Can you work these out from the model? Positions are in its coordinate system, mm. Give positions to 0.01 mm unless a question says otherwise; leave off trailing zeros. Loops run counter-clockwise (first coordinate to the right, second up) from the corner with the lowest first, then second, coordinate; pieces in that order, holes last. Notation, with made-up numbers: M 4,64 L 30,64 A29 cw 30,88 Z; hole C 58.5,-28 d7. An arc over 180 degrees is marked long. Use CSV: the item, a comma, the result in double quotes.
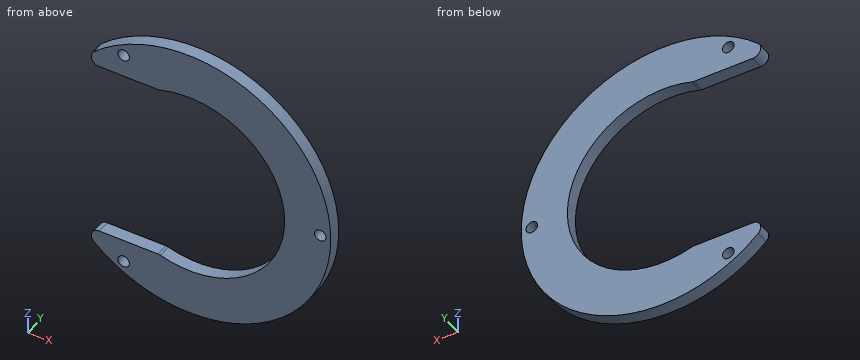
Autodesk Inventor part; units mm, degrees
ref_plane "YZ Plane" through (0, 0, 0) normal (1, 0, 0) x (0, 1, 0)
ref_plane "XZ Plane" through (0, 0, 0) normal (0, 1, 0) x (-1, 0, 0)
ref_plane "XY Plane" through (0, 0, 0) normal (0, 0, 1) x (1, 0, 0)
sketch "Sketch1" plane through (0, 0, 0) normal (0, 1, 0) x (-1, 0, 0)
  circle A0 centre (0, 0) radius 59
  circle A1 centre (0, 0) radius 81 construction
  circle A2 centre (0, 0) radius 87.5
  line L0 (90, -56) -> (10, -56)
  line L1 (10, -56) -> (10, 56)
  line L2 (10, 56) -> (90, 56)
  line L3 (90, 56) -> (90, -56)
  line L4 (90, -56) -> (10, 56) construction
  line L5 (10, -56) -> (90, 56) construction
  point P0 (50, 0)
  point P1 (90, 0)
  point P2 (10, 0)
  point P3 (60, -54.4151)
  point P4 (60, 54.4151)
  point P5 (80, 35.4436)
  point P6 (80, -35.4436)
  point P7 (67.2328, 56)
  point P8 (67.2328, -56)
  point P9 (18.5742, 56)
  point P10 (18.5742, -56)
  dimension "d0" = 118
  dimension "d1" = 162
  dimension "d2" = 175
  dimension "d7" = 112
  dimension "d9" = 80
  dimension "d10" = 10
extrude "Extrusion1" add sketch "Sketch1" along normal blind 8 contours A0 L0 A2 L2 picked at (48.009, -59.1067)
fillet "Fillet1" radius 5 4 edges at (-67.2328, 4, -56) (-67.2328, 4, 56) (-18.5742, 4, -56) (-18.5742, 4, 56)
sketch "Sketch2" plane through (0, 8, 0) normal (0, 1, 0) x (1, 0, 0)
  circle A0 centre (0, 0) radius 70.375
  line L0 (-36.4414, 79.1184) -> (-50.2978, 71.1184)
  line L1 (-50.2978, 71.1184) -> (-44.9056, 61.7788)
  arc A1 (-31.0492, 69.7788) -> (-44.9056, 61.7788) centre (0, 0) ccw
  line L2 (-31.0492, 69.7788) -> (-36.4414, 79.1184)
  circle A2 centre (-40.5, 70.1481) radius 3.5625
  circle A3 centre (-40.5, 70.1481) radius 3.5625
  line L3 (86.7392, -8) -> (86.7392, 8)
  line L4 (86.7392, 8) -> (75.9549, 8)
  arc A4 (75.9549, -8) -> (75.9549, 8) centre (0, 0) ccw
  line L5 (75.9549, -8) -> (86.7392, -8)
  arc A5 (80.9215, -3.5651) -> (80.9217, -3.5616) centre (0, 0) ccw
  arc A6 (81.0783, -3.5616) -> (80.9217, -3.5616) centre (81, 0) ccw
  line L6 (81.0783, -3.5616) -> (80.9215, -3.5651)
  line L7 (-50.2978, -71.1184) -> (-36.4414, -79.1184)
  line L8 (-36.4414, -79.1184) -> (-31.0492, -69.7788)
  arc A7 (-44.9056, -61.7788) -> (-31.0492, -69.7788) centre (0, 0) ccw
  line L9 (-44.9056, -61.7788) -> (-50.2978, -71.1184)
  circle A8 centre (-40.5, -70.1481) radius 3.5625
  point P0 (-65.1143, 450.6181)
extrude "Extrusion2" cut sketch "Sketch2" against normal blind 10 contours A2 | A5 A6 L6 | A8
properties part number "Cylinder Segment Holder" material "Acetal Resin, Black"
Q1. I want a section at C-C, the plane y = 4.25. State how many separate pieces and enclosed holes the cut face has, then the cut area to 3 significant figures.
Model answer:
separate pieces,"1"
enclosed holes,"3"
area,"9,250 mm2"
Q2. Please list where these lines run through material, in increasing order: L1, parallel to Z at x = 0, y = 4.75; L2, parallel to Z at x = -40.5, y = 4.25; L3, parallel to Z at x = -42, y = 5.5. Write a range as from..to.
Model answer:
L1,"-87.5..-59, 59..87.5"
L2,"-77.56..-73.71, -66.59..-56, 56..66.59, 73.71..77.56"
L3,"-76.76..-73.38, -66.92..-56, 56..66.92, 73.38..76.76"
Q3. I'm going to push flat-ended pins straight in: P1, Ø2, axis at y = 5, z = -31.5, coming from the +X side; P2, Ø2, axis at y = 1.5, z = 29, coming from the +X side; P3, Ø2, axis at y = 4.5, z = 58, coming from the +X side. Where does each tip first touch, or does it pass through?
Model answer:
P1,"x = 82.01"
P2,"x = 82.9"
P3,"x = 66.39"
Q4. I want a section at A-A, the plane x = 0. Please give me the cut outline in (y, z).
Model answer:
outline,"M 0,-87.5 L 8,-87.5 L 8,-59 L 0,-59 Z; M 0,59 L 8,59 L 8,87.5 L 0,87.5 Z"
Q5. I want a section at D-D, the plane x = -40.5. Please give me the cut outline in (y, z).
Model answer:
outline,"M 0,-77.56 L 8,-77.56 L 8,-73.71 L 0,-73.71 Z; M 0,-66.59 L 8,-66.59 L 8,-56 L 0,-56 Z; M 0,56 L 8,56 L 8,66.59 L 0,66.59 Z; M 0,73.71 L 8,73.71 L 8,77.56 L 0,77.56 Z"
Q6. I want a section at B-B, the plane z = 0. Please give me the cut outline in (x, y), then the cut area to 3 significant figures.
Model answer:
outline,"M 59,0 L 77.44,0 L 77.44,8 L 59,8 Z; M 84.56,0 L 87.5,0 L 87.5,8 L 84.56,8 Z"
area,"171 mm2"
